```python
from build123d import *

# Parameters (mm, degrees)
F0_W           = 100
F0_H           = 106
F0_R           = 2.5
F1_DEPTH       = 3
F2_R           = 3
F4_DEPTH       = 28
F5_DEPTH       = 20
F3_W           = 3
F3_H           = 15
F6_DEPTH       = 28
F7_DEPTH       = 15
F7_DEPTH_BACK  = 62
F9_DEPTH       = 20
F9_DEPTH_BACK  = 72
F11_DEPTH      = 20
F11_DEPTH_BACK = 72
F12_R          = 3.05
F13_R          = 3.05
F14_DEPTH      = 47
F15_R          = 3.05
F16_DEPTH      = 3
F16_DEPTH_BACK = 89
F17_DEPTH      = 2


with BuildPart() as f1:
    # F0 (on Top) → F1 (new body)
    with BuildSketch(Plane.XY):
        Rectangle(F0_W, F0_H)
        with Locations((-33.1323798252, -43.9004032683)):
            Circle(F0_R, mode=Mode.SUBTRACT)
        with Locations((33.1323798252, -43.9004032683)):
            Circle(F0_R, mode=Mode.SUBTRACT)
        with Locations((-33.1323798252, 43.9004032683)):
            Circle(F0_R, mode=Mode.SUBTRACT)
        with Locations((33.1323798252, 43.9004032683)):
            Circle(F0_R, mode=Mode.SUBTRACT)
    extrude(amount=F1_DEPTH)

    # F2
    f2_edges = [f1.edges().sort_by_distance(p)[0] for p in [
        (-50, -53, 1.5),
        (-50, 53, 1.5),
        (50, 53, 1.5),
        (50, -53, 1.5),
    ]]
    fillet(f2_edges, radius=F2_R)

    # F3 (on Top) → F4 (join)
    with BuildSketch(Plane.XY):
        Polygon((-23, -20.5), (-43, -20.5), (-43, -23.5), (-40, -23.5), (-26, -23.5), (-23, -23.5), align=None)
        Polygon((-43, 23.5), (-43, 20.5), (-23, 20.5), (-23, 23.5), (-26, 23.5), (-40, 23.5), align=None)
        Polygon((23, 20.5), (43, 20.5), (43, 23.5), (40, 23.5), (26, 23.5), (23, 23.5), align=None)
        Polygon((43, -23.5), (43, -20.5), (23, -20.5), (23, -23.5), (26, -23.5), (40, -23.5), align=None)
    extrude(amount=-F4_DEPTH)

    # F3 (on Top) → F5 (join)
    with BuildSketch(Plane.XY):
        Polygon((43, 20.5), (43, -20.5), (43, -23.5), (46, -23.5), (46, 23.5), (43, 23.5), align=None)
        Polygon((-43, -20.5), (-43, 20.5), (-43, 23.5), (-46, 23.5), (-46, -23.5), (-43, -23.5), align=None)
    extrude(amount=-F5_DEPTH)

    # F3 (on Top) → F6 (join)
    with BuildSketch(Plane.XY):
        with Locations((-41.5, 31)):
            Rectangle(F3_W, F3_H)
        with Locations((-24.5, 31)):
            Rectangle(F3_W, F3_H)
        with Locations((24.5, 31)):
            Rectangle(F3_W, F3_H)
        with Locations((41.5, 31)):
            Rectangle(F3_W, F3_H)
        with Locations((-41.5, -31)):
            Rectangle(F3_W, F3_H)
        with Locations((-24.5, -31)):
            Rectangle(F3_W, F3_H)
        with Locations((24.5, -31)):
            Rectangle(F3_W, F3_H)
        with Locations((41.5, -31)):
            Rectangle(F3_W, F3_H)
    extrude(amount=-F6_DEPTH)

    # F7 (add, two sides): faces of the model
    f7_faces = [f1.faces().sort_by_distance(p)[0] for p in [
        (-44.5, -23.5, -10),
        (44.5, -23.5, -10),
    ]]
    extrude(f7_faces, amount=F7_DEPTH)
    extrude(f7_faces, amount=-F7_DEPTH_BACK)

    # F8 (on face) → F9 (cut, two sides)
    with BuildSketch(Plane(origin=(-26, 0, 0), x_dir=(0, -1, 0), z_dir=(-1, 0, 0))) as f9_sk:
        Polygon((-23.5, -28), (-38.5, 0), (-38.5, -28), align=None)
    extrude(amount=F9_DEPTH, mode=Mode.SUBTRACT)
    extrude(f9_sk.sketch, amount=-F9_DEPTH_BACK, mode=Mode.SUBTRACT)

    # F10 (on face) → F11 (cut, two sides)
    with BuildSketch(Plane(origin=(-26, 0, 0), x_dir=(0, -1, 0), z_dir=(-1, 0, 0))) as f11_sk:
        Polygon((38.5, 0), (23.5, -28), (38.5, -28), align=None)
    extrude(amount=F11_DEPTH, mode=Mode.SUBTRACT)
    extrude(f11_sk.sketch, amount=-F11_DEPTH_BACK, mode=Mode.SUBTRACT)

    # F12 (on face) + F13 (on face) → F14 (cut, through all)
    with BuildSketch(Plane(origin=(0, 23.5, 0), x_dir=(-1, 0, 0), z_dir=(0, 1, 0))):
        with Locations((33, -23)):
            Circle(F12_R)
        with Locations((33, -9)):
            Circle(F12_R)
    with BuildSketch(Plane(origin=(0, 23.5, 0), x_dir=(-1, 0, 0), z_dir=(0, 1, 0))):
        with Locations((-33, -9)):
            Circle(F13_R)
        with Locations((-33, -23)):
            Circle(F13_R)
    extrude(amount=-F14_DEPTH, mode=Mode.SUBTRACT)

    # F15 (on face) → F16 (cut, two sides)
    with BuildSketch(Plane.YZ.offset(-43)) as f16_sk:
        with Locations((10.5, -10)):
            Circle(F15_R)
        with Locations((-10.5, -10)):
            Circle(F15_R)
    extrude(amount=-F16_DEPTH, mode=Mode.SUBTRACT)
    extrude(f16_sk.sketch, amount=F16_DEPTH_BACK, mode=Mode.SUBTRACT)

    # F17 (add): faces of the model
    f17_faces = [f1.faces().sort_by_distance(p)[0] for p in [
        (33, -22, -28),
        (-33, -22, -28),
        (-33, 22, -28),
        (33, 22, -28),
    ]]
    extrude(f17_faces, amount=F17_DEPTH)


solid = f1.part
```
Input: part model. Units: mm. Frame: model coordinates. A direction names the side the tool comes from. Coordinates: 2 decimals unless noted, no trailing zeros. Loops run counter-clockwise (first coordinate to the right, second up) from the corner with the lowest first, then second, coordinate; pieces in that order, holes last. Notation, with made-up numbers: (-19.5, 53) - (9.5, 53) arc R28 cw to (9.5, 87) - close; hole circle Ø11 at (16, 35.5). An arc over 180 degrees is marked (long way). Answer in a Markdown table with one row per item.
(1) Cut plane A-A on y = 10.5. Output: boundary loops of the cut face in (x, z).
Model answer:
| item | result |
|---|---|
| outline | (-50, 0) - (-46, 0) - (-46, -6.95) - (-43, -6.95) - (-43, 0) - (43, 0) - (43, -6.95) - (46, -6.95) - (46, 0) - (50, 0) - (50, 3) - (-50, 3) - close; (-46, -20) - (-43, -20) - (-43, -13.05) - (-46, -13.05) - close; (43, -20) - (46, -20) - (46, -13.05) - (43, -13.05) - close |
(2) Cut plane D-D on x = -33. Count the separate pieces of the cut face and the enclosed holes in it, plus the area to 3 significant figures.
Model answer:
| item | result |
|---|---|
| separate pieces | 7 |
| enclosed holes | 0 |
| area | 395 mm² |
(3) Mould query, pull axis X, two halves, no side actions, for faces 5 (the face through (-1, 1, 3)), 6 (the face through (-23, -28, -11)), 7 (the face through (46, -1, -10)). Classes: pulls with the +X half, pulls with the -X half, needs draft (parallel to the pull), parting line crosses it, or undercut.
Model answer:
| item | result |
|---|---|
| face 5 | needs draft |
| face 6 | undercut |
| face 7 | pulls with the +X half |
(4) Cut plane C-C on x = -19.5. Output: boundary loops of the cut face in (y, z), plus the area to 3 significant figures.
Model answer:
| item | result |
|---|---|
| outline | (-53, 0) - (53, 0) - (53, 3) - (-53, 3) - close |
| area | 318 mm² |
(5) Material intervals for L1, parallel to Z at x = 33, y = -22.3; L2, parallel to X at y = -31.5, z = -6.5; L3, parallel to X at y = 16, z = -10.5, sorted ascending. Write a range as from..to.
Model answer:
| item | result |
|---|---|
| L1 | z = -30..-26.05, -19.95..-12.05, -5.95..3 |
| L2 | x = -46..-40, -26..-23, 23..26, 40..46 |
| L3 | x = -46..-43, 43..46 |
(6) Set-up query: faces 1 (the face through (26, 29, -11)), 2 (the face through (-46, 1, -10)), 3 (the face through (-33, -20.5, -15)), 4 (the face through (-26, -28, -8)). Return all of +Z, -Z, +X, -X, +Y, -Y with unobstructed straight access to the full face (end or side cutting, diameter ignored); none if empty.
Model answer:
| item | result |
|---|---|
| face 1 | -Z, +Y |
| face 2 | -Z, -X, +Y, -Y |
| face 3 | -Z |
| face 4 | -Z, -Y |
(7) Pin query (flat end, axial travel): P1, Ø10, axis at x = -33, z = -23, coming from the -Y side; P2, Ø1.5, axis at x = -44, y = -13.5, coming from the -Z side; P3, Ø10, axis at y = 27.5, z = -16, coming from the -X side. Return the tip coordinate at first contact, or that it passes through.
Model answer:
| item | result |
|---|---|
| P1 | stops at y = -23.5 |
| P2 | stops at z = -20 |
| P3 | stops at x = -46 |
